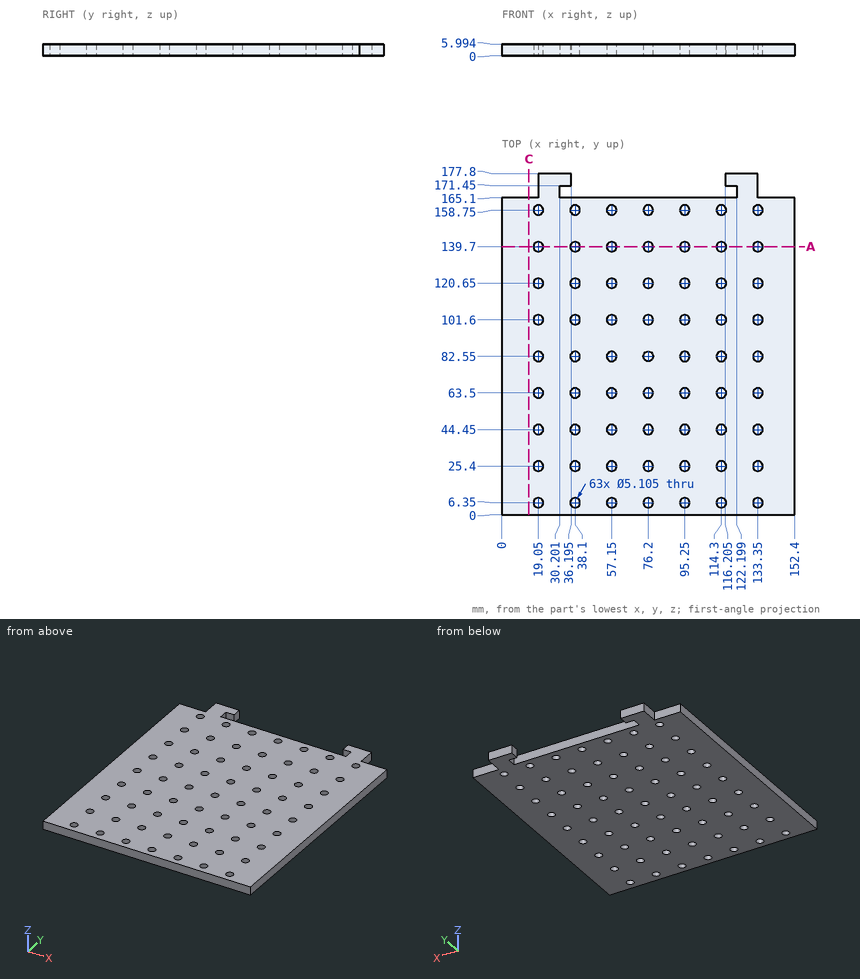
The figure shows three views and two pictorial views of one solid part (mm, origin at its lowest corner). Answer the questions. Round coordinates to 2 decimals unless told otherwise and drop trailing zeros. Write each loop counter-clockwise with the first axis right and the second up, starting at its lowest first coordinate (ties: lowest second). Pieces come first, ordered by that corner, then holes. Notation, with made-up numbers: (47, 71) - (90, 71) arc R14 ccw to (90, 84) - close; hole circle Ø4 at (43.5, 46.25). An arc over 180 degrees is marked (long way). One line per question, with ' | ' between items. Start each with the question number.
1. Find the intervals of material crossed by probe 1 along Y at (x, z) = (32.5, 3.9); probe 2 along Y at (x, z) = (111, 4.65), in increasing order. Write a range as [from, to].
2. Each of these flat-tipped pins is pushed along its axis until it touches: pin 1 (3 mm diameter, centred on y = 174, z = 4, fed in from -X); pin 2 (1.8 mm diameter, centred on x = 8.5, z = 3.5, fed in from +Y). Where does it stop, or does it pass through?
3. Section C-C (x = 14) is taken. Determine the outline of the cut face in (y, z) (1 decimal).
4. Section A-A (y = 139.7) is taken. Give the number of separate pieces and of enclosed holes in the cut face.
Filled in:
1) probe 1: [0, 165.1], [171.45, 177.8] | probe 2: [0, 165.1]
2) pin 1: x = 19.05 | pin 2: y = 165.1
3) outline: (0, 0) - (165.1, 0) - (165.1, 6) - (0, 6) - close
4) separate pieces: 8 | enclosed holes: 0
